Build history of the part. All positions in model axes, mm. Coordinates: 2 decimals unless noted, no trailing zeros. Order: outer loops, then holes, each group sorted by start corner. A loop starts at its lowest first (then second) coordinate and runs counter-clockwise, first axis right, second up. Notation, with made-up numbers: (4, 27) - (63, 27) arc R24 ccw to (63, 63) - close; hole circle Ø3 at (-19.5, -2). An arc over 180 degrees is marked (long way). One line per item, written item: value.
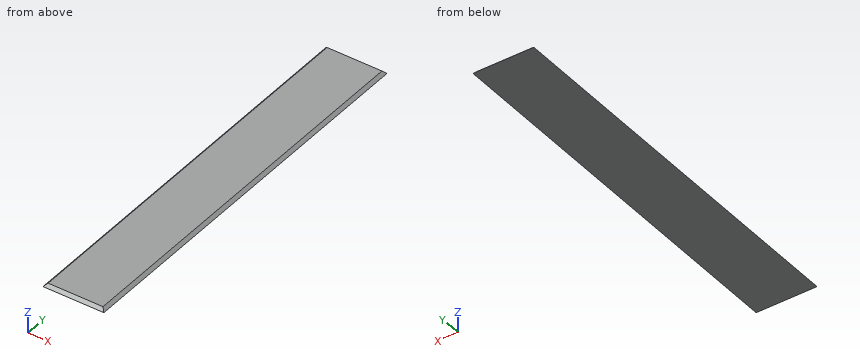
from build123d import *

# Parameters (mm, degrees)
F0_W     = 245
F0_H     = 1600
F1_DEPTH = 12
F2_SIZE  = 11.99999


# Not quite as in the source:
# - a fillet or chamfer is up to 0.001 mm smaller than in the source, because OpenCascade refuses the exact size


with BuildPart() as f1:
    # F0 (on Top) → F1 (new body)
    with BuildSketch(Plane.XY):
        Rectangle(F0_W, F0_H)
    extrude(amount=-F1_DEPTH)

    # F2 (size 12 in the source; OpenCascade refuses exactly that, so slightly less here)
    f2_edges = [f1.edges().sort_by_distance(p)[0] for p in [
        (0, -800, 0),
        (122.5, 0, 0),
        (-122.5, 0, 0),
        (0, 800, 0),
    ]]
    chamfer(f2_edges, length=F2_SIZE)


solid = f1.part
1. Flat gauge pins, fed straight in: P1, Ø5, axis at x = -11, z = -9, coming from the +Y side; P2, Ø5, axis at x = -31, z = -5.5, coming from the -Y side; P3, Ø3, axis at y = 309.5, z = -2.5, coming from the -X side. Where does each tip first touch, or does it go through?
Values found:
P1: stops at y = 799.5
P2: stops at y = -796
P3: stops at x = -114.5
2. Band-saw the part on B-B, the plane z = -2.5. Give the cut face in (x, y).
Values found:
outline: (-113, -790.5) - (113, -790.5) - (113, 790.5) - (-113, 790.5) - close
3. Probe line 1 along Y through (x, z) = (55.5, -11.25); line 2 along X through (y, z) = (406, -4); line 3 along X through (y, z) = (305.5, -10.5). List the from-to ranges inside material, lowest first.
Values found:
line 1: y = -799.25 to 799.25
line 2: x = -114.5 to 114.5
line 3: x = -121 to 121
